```python
from build123d import *

# Parameters (mm, degrees)
F4_DEPTH      = 5
F4_DEPTH_BACK = 5
F1_R          = 2
F5_DEPTH      = 12
F5_DEPTH_BACK = 25
F6_START      = 2.5
F6_DEPTH      = 3.5
F7_START      = -2
F3_R          = 2.25
F7_DEPTH      = 23


with BuildPart() as f4:
    # F0 (on Front) → F4 (new body, two sides)
    with BuildSketch(Plane.XZ) as f4_sk:
        with BuildLine():
            ThreePointArc((-2.0155644371, 1), (-0.3638449939, 2.2203866376), (1.5909902577, 1.5909902577))
            Line((1.5909902577, 1.5909902577), (1.5909902577, -1.5909902577))
            ThreePointArc((1.5909902577, -1.5909902577), (-0.3638449939, -2.2203866376), (-2.0155644371, -1))
            Line((-2.0155644371, -1), (-12, -1))
            Line((-12, -1), (-12, -5))
            Line((-12, -5), (0, -5))
            ThreePointArc((0, -5), (5, 0), (0, 5))
            Line((0, 5), (-37.0942321046, 5))
            Line((-37.0942321046, 5), (-39.0942321046, 8.4641016151))
            ThreePointArc((-39.0942321046, 8.4641016151), (-39.7165987233, 4.753081722), (-39.9874980463, 1))
            Line((-39.9874980463, 1), (-2.0155644371, 1))
        make_face()
    extrude(amount=F4_DEPTH)
    extrude(f4_sk.sketch, amount=-F4_DEPTH_BACK)

    # F1 (on Top) → F5 (cut, two sides)
    with BuildSketch(Plane.XY) as f5_sk:
        with Locations((-6, 0)):
            Circle(F1_R)
    extrude(amount=-F5_DEPTH, mode=Mode.SUBTRACT)
    extrude(f5_sk.sketch, amount=F5_DEPTH_BACK, mode=Mode.SUBTRACT)

    # F2 (on Top) → F6 (cut)
    with BuildSketch(Plane.XY.offset(F6_START)):
        Polygon((-4.2679491924, -3), (-2.5358983849, 0), (-4.2679491924, 3), (-7.7320508076, 3), (-9.4641016151, 0), (-7.7320508076, -3), align=None)
    extrude(amount=F6_DEPTH, mode=Mode.SUBTRACT)

    # F3 (on Front) → F7 (cut)
    with BuildSketch(Plane.XZ.offset(F7_START)):
        Circle(F3_R)
    extrude(amount=-F7_DEPTH, mode=Mode.SUBTRACT)


solid = f4.part
```
Verification items for the finished model (mm, model axes). A direction names the side the tool comes from. Coordinates: 2 decimals unless noted, no trailing zeros. Loops run counter-clockwise (first coordinate to the right, second up) from the corner with the lowest first, then second, coordinate; pieces in that order, holes last. Notation, with made-up numbers: (10.5, 21) - (46.5, 21) arc R23 cw to (46.5, 47) - close; hole circle Ø8 at (-5, 43). An arc over 180 degrees is marked (long way). Answer as a JSON object with one key per item and string values.
(1) Cross-section at D-D, the plane y = 0.75. Record the boundary of the cut face in (x, z).
Response:
{"outline": "(-39.99, 1) - (-7.85, 1) - (-7.85, 2.5) - (-9.03, 2.5) - (-9.03, 5) - (-37.09, 5) - (-39.09, 8.46) arc R40 ccw to start; (-12, -5) - (-7.85, -5) - (-7.85, -1) - (-12, -1) - close; (-4.15, -5) - (0, -5) arc R5 ccw to (0, 5) - (-2.97, 5) - (-2.97, 2.5) - (-4.15, 2.5) - (-4.15, 1) - (-2.02, 1) arc R2.25 cw to (1.59, 1.59) - (1.59, -1.59) arc R2.25 cw to (-2.02, -1) - (-4.15, -1) - close"}
(2) Mould release check, pull along Z, two halves, no side actions. Record for faces 1 (the flat face through (-5, 2, 2.5)), 2 (the flat face through (-6, 3, 4)), 3 (the flat face through (1.591, -2, 0)): pulls with the +Z half, pulls with the -Z half, needs draft (parallel to the pull), parting line crosses it, or undercut.
Response:
{"face 1": "pulls with the +Z half", "face 2": "needs draft", "face 3": "undercut"}
(3) Cross-section at C-C, the plane z = 0. Record the boundary of the cut face in (x, y), then the cut area to 3 significant figures.
Response:
{"outline": "(1.59, -5) - (5, -5) - (5, 5) - (2.25, 5) - (2.25, 2) - (1.59, 2) - close", "area": "32.1 mm²"}
(4) Cross-section at A-A, the plane x = -6. Record the boundary of the cut face in (y, z), then the cut area to 3 significant figures.
Response:
{"outline": "(-5, -5) - (-2, -5) - (-2, -1) - (-5, -1) - close; (-5, 1) - (-2, 1) - (-2, 2.5) - (-3, 2.5) - (-3, 5) - (-5, 5) - close; (2, -5) - (5, -5) - (5, -1) - (2, -1) - close; (2, 1) - (5, 1) - (5, 5) - (3, 5) - (3, 2.5) - (2, 2.5) - close", "area": "43.0 mm²"}
(5) Access from +Z, -Z, +X, -X, +Y, -Y to the whole of each face (thin tool, end or side, straight path). Record for faces 4 (the flat face through (-13, -5, 2)), 5 (the flat face through (-8, 1, -1)), 6 (the flat face through (-18, 0, 5)), 7 (the flat face through (-8.6, -1.5, 3.7)).
Response:
{"face 4": "+Z, -Z, +X, -X, -Y", "face 5": "-X, +Y, -Y", "face 6": "+Z, +X, +Y, -Y", "face 7": "+Z"}
(6) Cross-section at B-B, the plane y = 4. Record the boundary of the cut face in (x, z).
Response:
{"outline": "(-39.99, 1) - (-2.02, 1) arc R2.25 cw (long way) to (-2.02, -1) - (-12, -1) - (-12, -5) - (0, -5) arc R5 ccw to (0, 5) - (-37.09, 5) - (-39.09, 8.46) arc R40 ccw to start"}
(7) Scan lines: line 1 along Y through (x, z) = (-6, 2.05); line 2 along X through (y, z) = (0, 1.8); line 3 along X through (y, z) = (0, 1.55). Record each from-to range of solid material in increasing order.
Response:
{"line 1": "y = -5 to -2, 2 to 5", "line 2": "x = -39.96 to -8, -4 to -1.35, 1.35 to 4.66", "line 3": "x = -39.97 to -8, -4 to -1.63, 1.59 to 4.75"}
(8) Go/stop test with flat-tipped pins: pin 1 Ø6 at (x, y) = (-34, 3) entering from +Z; pin 2 Ø3 at (x, y) = (-6, -1) entering from +Z; pin 3 Ø1.2 at (y, z) = (-2, -2.5) entering from -X. Record where each tip stops, or that it passes through.
Response:
{"pin 1": "stops at z = 5", "pin 2": "stops at z = 2.5", "pin 3": "stops at x = -12"}
